from build123d import *

# Parameters (mm, degrees)
BOSS_EXTRUDE1_DEPTH            = 12.7
CUT_EXTRUDE1_DEPTH             = 13.7
SKETCH3_W                      = 18.5
SKETCH3_H                      = 12.7
F_3_7_3_7_DIAMETER_HOLE1_D     = 3.7
F_3_7_3_7_DIAMETER_HOLE1_DEPTH = 22.5
SKETCH6_W                      = 1.85
SKETCH6_H                      = 20.98
F_3_7_3_7_DIAMETER_HOLE3_D     = 3.7
F_3_7_3_7_DIAMETER_HOLE3_DEPTH = 44.98
FILLET1_R                      = 1.5
FILLET2_R                      = 6.35


with BuildPart() as part:
    # Sketch1 → Boss-Extrude1 (new body)
    with BuildSketch(Plane(origin=(0, 0, -12.299495873), x_dir=(-1, 0, 0), z_dir=(0, 0, -1))):
        with BuildLine():
            Line((24.859325054, -22.385915399), (24.859325054, 8.305102167))
            Line((24.859325054, 8.305102167), (9.793928734, 8.305102167))
            ThreePointArc((9.793928734, 8.305102167), (-15.308438691, 22.204357242), (-33.620674946, 0.114084601))
            Line((-33.620674946, 0.114084601), (-47.140674946, 0.114084601))
            Line((-47.140674946, 0.114084601), (-47.140674946, -22.385915399))
            Line((-47.140674946, -22.385915399), (24.859325054, -22.385915399))
        make_face()
    extrude(amount=-BOSS_EXTRUDE1_DEPTH)

    # Sketch2 → Cut-Extrude1 (cut, through all)
    with BuildSketch(Plane.XY.offset(0.400504127)):
        with BuildLine():
            Line((-24.859325054, 1.614084601), (-24.859325054, -1.385915399))
            Line((-24.859325054, -1.385915399), (-7.298413969, -1.385915399))
            ThreePointArc((-7.298413969, -1.385915399), (-7.359325054, 0.114084601), (-7.298413969, 1.614084601))
            Line((-7.298413969, 1.614084601), (-24.859325054, 1.614084601))
        make_face()
    extrude(amount=-CUT_EXTRUDE1_DEPTH, mode=Mode.SUBTRACT)

    # Sketch3 → Cut-Revolve1 (revolve, cut)
    with BuildSketch(Plane.XZ.offset(-0.114084601)):
        with Locations((20.390674946, -5.949495873)):
            Rectangle(SKETCH3_W, SKETCH3_H)
    revolve(axis=Axis((11.140674946, 0.114084601, 0.400504127), (0, 0, -1)), mode=Mode.SUBTRACT)

    # Ø3.7 (3.7) Diameter Hole1
    with Locations(Plane(origin=(0, 0.114084601, 0), x_dir=(1, 0, 0), z_dir=(0, 1, 0))):
        with Locations((43.140674946, 5.949495873)):
            Hole(F_3_7_3_7_DIAMETER_HOLE1_D / 2, depth=F_3_7_3_7_DIAMETER_HOLE1_DEPTH)

    # Sketch6 → Ø3.7 (3.7) Diameter Hole2 (revolve, cut)
    with BuildSketch(Plane(origin=(-20.859325054, 1.614084601, -5.949495873), x_dir=(0, 0, -1), z_dir=(1, 0, 0))):
        with Locations((0.925, 10.49)):
            Rectangle(SKETCH6_W, SKETCH6_H)
    revolve(axis=Axis((-20.859325054, -4.735915399, -5.949495873), (0, 1, 0)), mode=Mode.SUBTRACT)

    # Ø3.7 (3.7) Diameter Hole3
    with Locations(Plane(origin=(0, -22.385915399, 0), x_dir=(-1, 0, 0), z_dir=(0, -1, 0))):
        with Locations((20.859325054, 5.949495873)):
            Hole(F_3_7_3_7_DIAMETER_HOLE3_D / 2, depth=F_3_7_3_7_DIAMETER_HOLE3_DEPTH)

    # Fillet1
    fillet1_edges = [part.edges().sort_by_distance(p)[0] for p in [
        (47.140674946, 0.114084601, -5.949495873),
        (-24.859325054, 8.305102167, -5.949495873),
    ]]
    fillet(fillet1_edges, radius=FILLET1_R)

    # Fillet2
    fillet2_edges = [part.edges().sort_by_distance(p)[0] for p in [
        (33.620674946, 0.114084601, -5.949495873),
        (-9.793928734, 8.305102167, -5.949495873),
    ]]
    fillet(fillet2_edges, radius=FILLET2_R)


solid = part.part
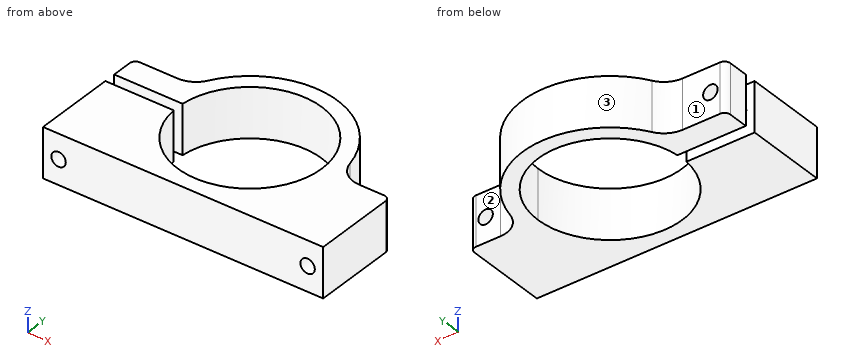
The model under review builds one solid part; all positions refer to its coordinate system, in mm. Face numbers are marked on the shaded views. A direction names the side the tool comes from. Round coordinates to 2 decimals unless told otherwise and drop trailing zeros. Loops run counter-clockwise (first coordinate to the right, second up) from the corner with the lowest first, then second, coordinate; pieces in that order, holes last. Notation, with made-up numbers: M -34,43.5 L 24,43.5 A27 cw 24,69.5 Z; hole C 78,16.25 d1. An arc over 180 degrees is marked long. Answer as CSV lines item,"result".
1. We need section A-A (y = -2.5). Give the boundary of the cut face in (x, z).
Outcome:
outline,"M -24.86,-12.3 L -7.17,-12.3 L -7.17,0.4 L -24.86,0.4 Z; M 29.46,-12.3 L 47.14,-12.3 L 47.14,0.4 L 29.46,0.4 Z; hole C -20.86,-5.95 d3.7; hole C 43.14,-5.95 d3.7"
2. To check wall thickness, follow L1, parallel to Y at x = -19, z = -3; L2, parallel to X at y = -15.5, z = -7.25; L3, parallel to X at y = -15, z = -5.5. State the ranges of each line that lie inside material, in increasing order. Write a range as [from, to].
Outcome:
L1,"y = [-22.39, -1.39], [1.61, 8.31]"
L2,"x = [-24.86, -22.18], [-19.54, 1.22], [21.06, 41.82], [44.46, 47.14]"
L3,"x = [-24.86, -22.65], [-19.06, 0.47], [21.81, 41.35], [44.94, 47.14]"
3. We need section C-C (y = 6). Give the boundary of the cut face in (x, z).
Outcome:
outline,"M -24.86,-12.3 L -6.4,-12.3 L -6.4,0.4 L -24.86,0.4 Z; M 28.68,-12.3 L 32.84,-12.3 L 32.84,0.4 L 28.68,0.4 Z; hole C -20.86,-5.95 d3.7"
4. We need section D-D (z = -7). Give the boundary of the cut face in (x, y), plus the area to 3 significant figures.
Outcome:
outline,"M -24.86,-22.39 L -22.38,-22.39 L -22.38,-1.39 L -24.86,-1.39 Z; M -24.86,1.61 L -22.38,1.61 L -22.38,8.31 L -23.36,8.31 A1.5 ccw -24.86,6.81 Z; M -19.34,-22.39 L 41.62,-22.39 L 41.62,0.11 L 39.26,0.11 A6.35 cw 33.07,5.07 A22.48 ccw -8.27,11.45 A6.35 cw -13.75,8.31 L -19.34,8.31 L -19.34,1.61 L -7.3,1.61 A18.5 cw long -7.3,-1.39 L -19.34,-1.39 Z; M 44.66,-22.39 L 47.14,-22.39 L 47.14,-1.39 A1.5 ccw 45.64,0.11 L 44.66,0.11 Z"
area,"1,260 mm2"
5. For the marked faces 1, 2 and 3, list the 3-axis set-ups (+Z, -Z, +X, -X, +Y, -Y) from which the entire face can be reached by the end or side of a thin tool; tool diameter is ignored.
Outcome:
face 1,"+Z, -Z, -X, +Y"
face 2,"+Z, -Z, +X, +Y"
face 3,"+Z, -Z, +Y"
6. We need section B-B (x = 9). Give the boundary of the cut face in (y, z), plus the area to 3 significant figures.
Outcome:
outline,"M -22.39,-12.3 L -18.26,-12.3 L -18.26,0.4 L -22.39,0.4 Z; M 18.49,-12.3 L 22.49,-12.3 L 22.49,0.4 L 18.49,0.4 Z"
area,"103 mm2"
7. Insertion check: pin 1 Ø6 at (x, z) = (-20.86, -5.95) entering from +Y; pin 2 Ø3 at (x, z) = (43, -9) entering from +Y; pin 3 Ø3.5 at (x, z) = (43.14, -5.95) entering from +Y; pin 4 Ø6 at (x, z) = (29, -10) entering from +Y. Each pin has a flat end and moves straight along its axis. Give the tip position at first contact, or say it passes through.
Outcome:
pin 1,"stops at y = 8.31"
pin 2,"stops at y = 0.11"
pin 3,"passes through"
pin 4,"stops at y = 16.98"
